Input: part model. Units: mm. Frame: model coordinates. A direction names the side the tool comes from. Coordinates: 2 decimals unless noted, no trailing zeros. Write each loop counter-clockwise with the first axis right and the second up, starting at its lowest first coordinate (ties: lowest second). Pieces come first, ordered by that corner, then holes. Notation, with made-up numbers: (-17, 69.5) - (18, 69.5) arc R19 cw to (18, 94.5) - close; hole circle Ø2 at (35, 82). An arc over 180 degrees is marked (long way). Use a Markdown table: item, result. Add a question column.
Q1. Pin query (flat end, axial travel): P1, Ø0.5, axis at y = 0.5, z = -7.5, coming from the -X side; P2, Ø10, axis at x = 22, z = 11, coming from the +Y side; P3, Ø1.5, axis at x = 8.5, y = 1.5, coming from the -Z side; P4, Ø4, axis at x = 24, y = 7.5, coming from the +Z side. Return the tip coordinate at first contact, or that it passes through.
Q2. Set-up query: faces 4 (the face through (28.25, 0.5, -7.8)), 5 (the face through (36.5, 1.5, 15.5)), 6 (the face through (0, 5, -3)), 7 (the face through (36.5, 8, 34)), 8 (the face through (28.25, 5, -4)). Return all of +Z, -Z, +X, -X, +Y, -Y with unobstructed straight access to the full face (end or side cutting, diameter ignored); none if empty.
Q3. Section query D-D (x = 35.5). Return the cut outline in (y, z).
Q4. Mould query, pull axis Z, two halves, no side actions, for faces 1 (the face through (31.5, 8, 34)), 2 (the face through (34, 2, 15)), 3 (the face through (29, 5, -6)). Classes: released by +Z, released by -Z, zero draft, split by the parting line, or undercut.
Q5. Section query B-B (y = 8.25). Return the cut outline in (x, z).
Q6. Material intervals for probe 1 along Y at (x, z) = (20.5, -4); probe 2 along X at (y, z) = (1.75, -2); probe 3 along Y at (x, z) = (31, 32), sorted ascending. Write a range as from..to.
Q7. Section query A-A (y = 5). Return the cut outline in (x, z), then the cut area to 4 significant figures.
Q8. Section query C-C (z = 13). Return the cut outline in (x, y), then the cut area to 3 significant figures.
from build123d import *

# Parameters (mm, degrees)
BOSS_EXTRUDE1_DEPTH = 9
SKETCH2_W           = 8
SKETCH2_H           = 36.5
CUT_EXTRUDE2_DEPTH  = 7
SKETCH3_W           = 1.5
SKETCH3_H           = 36.5
CUT_EXTRUDE3_DEPTH  = 1
SKETCH4_W           = 1.75
SKETCH4_H           = 3
CUT_EXTRUDE4_DEPTH  = 53.440442409
SKETCH5_W           = 5
SKETCH5_H           = 45
CUT_EXTRUDE5_DEPTH  = 1.5
CUT_EXTRUDE6_DEPTH  = 1
SKETCH7_W           = 20
SKETCH7_H           = 1.5
CUT_EXTRUDE7_DEPTH  = 53.440442409
SKETCH8_W           = 1.75
SKETCH8_H           = 3
CUT_EXTRUDE8_DEPTH  = 53.440442409


with BuildPart() as part:
    # Sketch1 → Boss-Extrude1 (new body)
    with BuildSketch(Plane(origin=(0, 0, 0), x_dir=(1, 0, 0), z_dir=(0, 1, 0))):
        Polygon((0, 0), (30, 0), (30, -35), (38, -35), (38, 10), (30, 10), (0, 5), align=None)
    extrude(amount=BOSS_EXTRUDE1_DEPTH)

    # Sketch2 → Cut-Extrude2 (cut)
    with BuildSketch(Plane(origin=(0, 9, 0), x_dir=(1, 0, 0), z_dir=(0, 1, 0))):
        with Locations((34, -15.25)):
            Rectangle(SKETCH2_W, SKETCH2_H)
    extrude(amount=-CUT_EXTRUDE2_DEPTH, mode=Mode.SUBTRACT)

    # Sketch3 → Cut-Extrude3 (cut)
    with BuildSketch(Plane(origin=(0, 2, 0), x_dir=(1, 0, 0), z_dir=(0, 1, 0))):
        with Locations((37.25, -15.25)):
            Rectangle(SKETCH3_W, SKETCH3_H)
        with Locations((30.75, -15.25)):
            Rectangle(SKETCH3_W, SKETCH3_H)
    extrude(amount=-CUT_EXTRUDE3_DEPTH, mode=Mode.SUBTRACT)

    # Sketch4 → Cut-Extrude4 (cut, through all)
    with BuildSketch(Plane(origin=(0, 9, 0), x_dir=(1, 0, 0), z_dir=(0, 1, 0))):
        with Locations((29.125, 1.5)):
            Rectangle(SKETCH4_W, SKETCH4_H)
    extrude(amount=-CUT_EXTRUDE4_DEPTH, mode=Mode.SUBTRACT)

    # Sketch5 → Cut-Extrude5 (cut)
    with BuildSketch(Plane(origin=(0, 9, 0), x_dir=(1, 0, 0), z_dir=(0, 1, 0))):
        with Locations((34, -12.5)):
            Rectangle(SKETCH5_W, SKETCH5_H)
    extrude(amount=-CUT_EXTRUDE5_DEPTH, mode=Mode.SUBTRACT)

    # Sketch6 → Cut-Extrude6 (cut)
    with BuildSketch(Plane(origin=(0, 0, 0), x_dir=(-1, 0, 0), z_dir=(0, -1, 0))):
        Polygon((-28.25, 0), (-28.25, 9.708333333), (0, 5), (0, 0), align=None)
    extrude(amount=-CUT_EXTRUDE6_DEPTH, mode=Mode.SUBTRACT)

    # Sketch7 → Cut-Extrude7 (cut, through all)
    with BuildSketch(Plane(origin=(0, 9, 0), x_dir=(1, 0, 0), z_dir=(0, 1, 0))):
        with Locations((18.25, 0.75)):
            Rectangle(SKETCH7_W, SKETCH7_H)
    extrude(amount=-CUT_EXTRUDE7_DEPTH, mode=Mode.SUBTRACT)

    # Sketch8 → Cut-Extrude8 (cut, through all)
    with BuildSketch(Plane(origin=(0, 9, 0), x_dir=(1, 0, 0), z_dir=(0, 1, 0))):
        with Locations((29.125, 4.5)):
            Rectangle(SKETCH8_W, SKETCH8_H)
    extrude(amount=-CUT_EXTRUDE8_DEPTH, mode=Mode.SUBTRACT)


solid = part.part
Values follow:
| question | item | result |
|---|---|---|
| 1 | P1 | x = 28.25 |
| 1 | P2 | through |
| 1 | P3 | z = -6.54 |
| 1 | P4 | z = -1.5 |
| 2 | face 4 | +Z, -Z, -X, -Y |
| 2 | face 5 | +X, +Y |
| 2 | face 6 | +Z, -Z, -X, +Y, -Y |
| 2 | face 7 | +Z, -Z, +Y |
| 2 | face 8 | +Z, +Y, -Y |
| 3 | outline | (0, -10) - (7.5, -10) - (7.5, -3) - (2, -3) - (2, 33.5) - (7.5, 33.5) - (7.5, 35) - (0, 35) - close |
| 4 | face 1 | zero draft |
| 4 | face 2 | undercut |
| 4 | face 3 | released by +Z |
| 5 | outline | (0, -5) - (30, -10) - (31.5, -10) - (31.5, -3) - (30, -3) - (30, -6) - (28.25, -6) - (28.25, -1.5) - (8.25, -1.5) - (8.25, 0) - (0, 0) - close; (30, 33.5) - (31.5, 33.5) - (31.5, 35) - (30, 35) - close; (36.5, -10) - (38, -10) - (38, -3) - (36.5, -3) - close; (36.5, 33.5) - (38, 33.5) - (38, 35) - (36.5, 35) - close |
| 6 | probe 1 | 1..9 |
| 6 | probe 2 | 0..28.25, 31.5..36.5 |
| 6 | probe 3 | 0..1 |
| 7 | outline | (0, -5) - (30, -10) - (38, -10) - (38, -3) - (30, -3) - (30, -6) - (28.25, -6) - (28.25, -1.5) - (8.25, -1.5) - (8.25, 0) - (0, 0) - close; (30, 33.5) - (38, 33.5) - (38, 35) - (30, 35) - close |
| 7 | area | 252.5 mm2 |
| 8 | outline | (30, 0) - (38, 0) - (38, 1) - (36.5, 1) - (36.5, 2) - (31.5, 2) - (31.5, 1) - (30, 1) - close |
| 8 | area | 13.0 mm2 |
